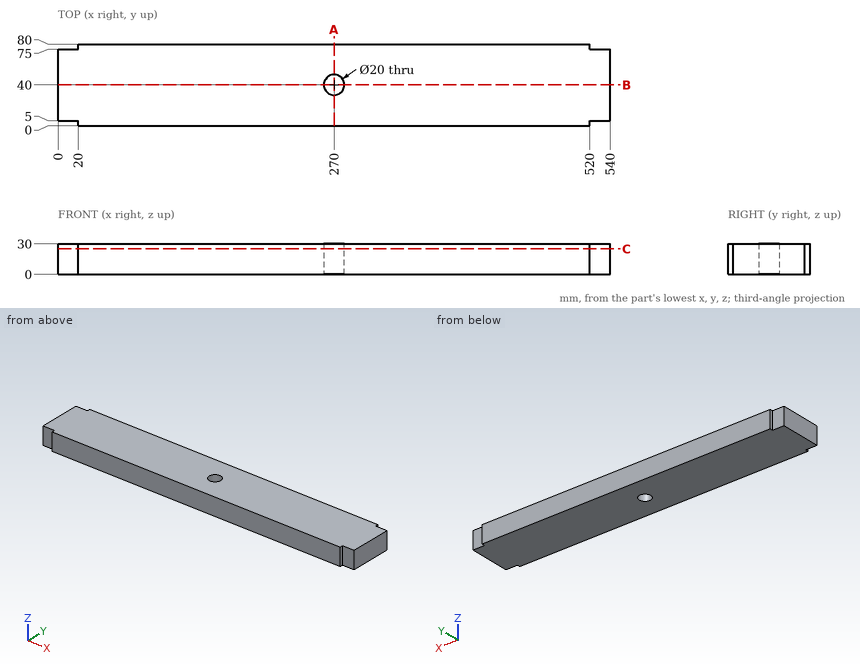
Design review of the part shown in the three views and the two pictorial views. Dimensions are in mm from the part's minimum x, y and z. Give positions to 0.01 mm unless a question says otherwise; leave off trailing zeros. Loops run counter-clockwise (first coordinate to the right, second up) from the corner with the lowest first, then second, coordinate; pieces in that order, holes last. Notation, with made-up numbers: M 82,62.5 L 127,62.5 A16 ccw 127,79.5 Z; hole C -27,44 d1. An arc over 180 degrees is marked long. Put each result on its own line as item: value. Start each with the question number.
(1) For pin 1 (2.5 mm diameter, centred on y = 77.5, z = 18, fed in from +X); pin 2 (10 mm diameter, centred on x = 12, z = 9.5, fed in from -Y); pin 3 (2.5 mm diameter, centred on y = 3, z = 9, fed in from -X), all flat-tipped, find the tip position at first contact; note any pin that passes through.
(2) Add section A-A, the plane x = 270. Write out the cut boundary in (y, z).
(3) Wall thickness on L1, parallel to Y at x = 270, z = 22.75; L2, parallel to X at y = 47, z = 23.75; L3, parallel to X at y = 37, z = 19.75: over which ranges is each line inside the solid? List them lowest first.
(4) Add section B-B, the plane y = 40. Write out the cut boundary in (x, z).
(5) Add section C-C, the plane z = 25. Write out the cut boundary in (x, y), then the cut area to 3 significant figures.
Result:
1. pin 1: stops at x = 520
1. pin 2: stops at y = 5
1. pin 3: stops at x = 20
2. outline: M 0,0 L 30,0 L 30,30 L 0,30 Z; M 50,0 L 80,0 L 80,30 L 50,30 Z
3. L1: y = 0 to 30, 50 to 80
3. L2: x = 0 to 262.86, 277.14 to 540
3. L3: x = 0 to 260.46, 279.54 to 540
4. outline: M 0,0 L 260,0 L 260,30 L 0,30 Z; M 280,0 L 540,0 L 540,30 L 280,30 Z
5. outline: M 0,5 L 20,5 L 20,0 L 520,0 L 520,5 L 540,5 L 540,75 L 520,75 L 520,80 L 20,80 L 20,75 L 0,75 Z; hole C 270,40 d20
5. area: 42,500 mm^2
